from build123d import *

# Parameters (mm, degrees)
F0_W      = 96
F0_H      = 64
F1_DEPTH  = 16
F3_DEPTH  = 16
F4_W      = 40
F4_H      = 28
F5_DEPTH  = 42
F7_DEPTH  = 42
F8_W      = 20
F8_H      = 16
F9_DEPTH  = 16
F11_DEPTH = 12


with BuildPart() as f1:
    # F0 (on Top) → F1 (new body)
    with BuildSketch(Plane.XY):
        with Locations((-41.832156, -7.992789)):
            Rectangle(F0_W, F0_H)
    extrude(amount=F1_DEPTH)

    # F2 (on face) → F3 (join)
    with BuildSketch(Plane(origin=(-89.832156, 0, 0), x_dir=(0, -1, 0), z_dir=(-1, 0, 0))):
        with BuildLine():
            Line((-24.007211, 64), (-24.007211, 16))
            Line((-24.007211, 16), (39.992789, 16))
            Line((39.992789, 16), (39.992789, 53.190336))
            ThreePointArc((39.992789, 53.190336), (29.165485, 61.172682), (16.014263, 64))
            Line((16.014263, 64), (-24.007211, 64))
        make_face()
    extrude(amount=-F3_DEPTH)

    # F4 (on face) → F5 (join)
    with BuildSketch(Plane(origin=(0, 24.007211, 0), x_dir=(-1, 0, 0), z_dir=(0, 1, 0))):
        with Locations((53.832156, 30)):
            Rectangle(F4_W, F4_H)
    extrude(amount=-F5_DEPTH)

    # F6 (on face) → F7 (cut)
    with BuildSketch(Plane.XZ.offset(17.992789)):
        with BuildLine():
            ThreePointArc((-65.832156, 44), (-53.832156, 32), (-41.832156, 44))
            Line((-41.832156, 44), (-65.832156, 44))
        make_face()
    extrude(amount=-F7_DEPTH, mode=Mode.SUBTRACT)

    # F8 (on face) → F9 (cut)
    with BuildSketch(Plane.XY.offset(16)):
        with Locations((-3.832156, -15.992789)):
            Rectangle(F8_W, F8_H)
        with BuildLine():
            ThreePointArc((-13.832156, -7.992789), (-21.832156, -15.992789), (-13.832156, -23.992789))
            Line((-13.832156, -23.992789), (-13.832156, -7.992789))
        make_face()
    extrude(amount=-F9_DEPTH, mode=Mode.SUBTRACT)

    # F10 (on face) → F11 (join)
    with BuildSketch(Plane(origin=(0, 24.007211, 0), x_dir=(-1, 0, 0), z_dir=(0, 1, 0))):
        Polygon((33.832156, 44), (-6.167844, 16), (33.832156, 16), align=None)
    extrude(amount=-F11_DEPTH)


solid = f1.part
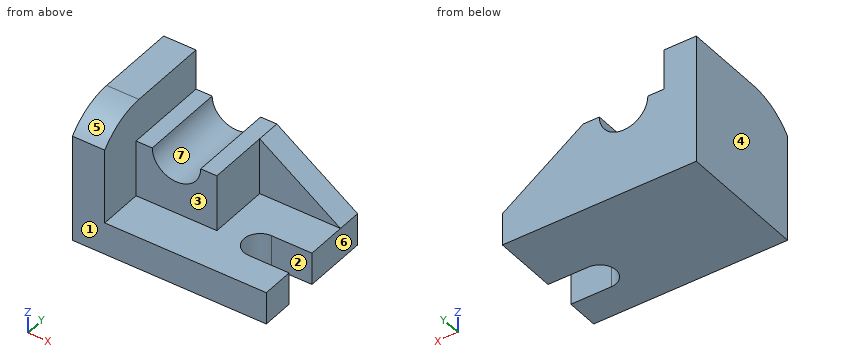
The model under review builds one solid part; all positions refer to its coordinate system, in mm. Face numbers are marked on the shaded views. A direction names the side the tool comes from. Coordinates: 2 decimals unless noted, no trailing zeros. Write each loop counter-clockwise with the first axis right and the second up, starting at its lowest first coordinate (ties: lowest second). Pieces come first, ordered by that corner, then holes. Notation, with made-up numbers: (24.5, -8.5) -> (46.5, -8.5) arc R24 ccw to (46.5, 6.5) -> close; hole circle Ø7 at (-27, 10). An arc over 180 degrees is marked (long way). Answer in a Markdown table with one row per item.
1. We need section A-A, the plane x = -2.5. State the section outline as (y, z) points.
Answers below:
| item | result |
|---|---|
| outline | (-39.99, 0) -> (-23.99, 0) -> (-23.99, 16) -> (-39.99, 16) -> close; (-7.99, 0) -> (24.01, 0) -> (24.01, 22.07) -> (12.01, 22.07) -> (12.01, 16) -> (-7.99, 16) -> close |
2. We need section C-C, the plane y = -10. State the section outline as (x, z) points.
Answers below:
| item | result |
|---|---|
| outline | (-89.83, 0) -> (-19.13, 0) -> (-19.13, 16) -> (-33.83, 16) -> (-33.83, 44) -> (-41.83, 44) arc R12 cw to (-65.83, 44) -> (-73.83, 44) -> (-73.83, 64) -> (-89.83, 64) -> close |
3. We need section B-B, the plane z = 35.5. State the section outline as (x, y) points, and give its area (3 significant figures).
Answers below:
| item | result |
|---|---|
| outline | (-89.83, -39.99) -> (-73.83, -39.99) -> (-73.83, -17.99) -> (-62.3, -17.99) -> (-62.3, 24.01) -> (-89.83, 24.01) -> close; (-45.36, -17.99) -> (-33.83, -17.99) -> (-33.83, 12.01) -> (-21.69, 12.01) -> (-21.69, 24.01) -> (-45.36, 24.01) -> close |
| area | 2,140 mm^2 |
4. Clearance check with flat-ended pins moving along their axes: pin 1 Ø14 at (x, z) = (-17.5, 31.5) entering from -Y; pin 2 Ø2.5 at (x, y) = (-71.5, 11.5) entering from +Z; pin 3 Ø12 at (x, y) = (-47.5, -22.5) entering from -Z; pin 4 Ø6 at (x, y) = (-27, 8) entering from +Z. State where each tip first meets the part, or that it passes through.
Answers below:
| item | result |
|---|---|
| pin 1 | stops at y = 12.01 |
| pin 2 | stops at z = 44 |
| pin 3 | stops at z = 0 |
| pin 4 | stops at z = 16 |
5. For the marked faces 1, 2 and 3, list the 3-axis set-ups (+Z, -Z, +X, -X, +Y, -Y) from which the entire face can be reached by the end or side of a thin tool; tool diameter is ignored.
Answers below:
| item | result |
|---|---|
| face 1 | +Z, -Z, +X, -X, -Y |
| face 2 | +Z, -Z, +X |
| face 3 | +Z, +X, -Y |
6. Wall thickness on probe 1 along X at (y, z) = (4.5, 43.5); probe 2 along X at (y, z) = (-32, 22); probe 3 along Y at (x, z) = (-66, 33): over which ranges is each line inside the solid? List them lowest first. Write a range as [from, to].
Answers below:
| item | result |
|---|---|
| probe 1 | x = [-89.83, -65.82], [-41.84, -33.83] |
| probe 2 | x = [-89.83, -73.83] |
| probe 3 | y = [-17.99, 24.01] |
7. Draft analysis for pull direction X (two halves, no side actions). For the marked faces 4, 5, 6 and 7, state which applies: +X half, -X half, draft (parallel to the pull), parting line (faces both ways), or undercut.
Answers below:
| item | result |
|---|---|
| face 4 | -X half |
| face 5 | draft |
| face 6 | +X half |
| face 7 | undercut |
8. We need section D-D, the plane x = -16. State the section outline as (y, z) points, and give its area (3 significant figures).
Answers below:
| item | result |
|---|---|
| outline | (-39.99, 0) -> (-23.69, 0) -> (-23.69, 16) -> (-39.99, 16) -> close; (-8.29, 0) -> (24.01, 0) -> (24.01, 31.52) -> (12.01, 31.52) -> (12.01, 16) -> (-8.29, 16) -> close |
| area | 964 mm^2 |
